from build123d import *
from OCP.BRepFilletAPI import BRepFilletAPI_MakeChamfer

# Parameters (mm, degrees)
PROFILE_SKETCH_W         = 14.3
PROFILE_SKETCH_H         = 6.7
PROFILE_SKETCH_W_2       = 10.1
PROFILE_SKETCH_H_2       = 2.5
PROFILE_EXTRUDE_DEPTH    = 15
OUTSIDE_CORNER_FILLETS_R = 1.5
END_1_CHAMFER_SIZE       = 1
END_1_CHAMFER_SIZE2      = 0.363970234
END_2_CHAMFER_SIZE       = 1
END_2_CHAMFER_SIZE2      = 0.363970234
TRANSITION_FILLETS_R     = 2.5


with BuildPart() as part:
    # Profile Sketch → Profile Extrude (new body)
    with BuildSketch(Plane.XY):
        Rectangle(PROFILE_SKETCH_W, PROFILE_SKETCH_H)
        Rectangle(PROFILE_SKETCH_W_2, PROFILE_SKETCH_H_2, mode=Mode.SUBTRACT)
    extrude(amount=PROFILE_EXTRUDE_DEPTH)

    # Outside Corner Fillets
    outside_corner_fillets_edges = [part.edges().sort_by_distance(p)[0] for p in [
        (7.15, -3.35, 7.5),
        (-7.15, -3.35, 7.5),
        (-7.15, 3.35, 7.5),
        (7.15, 3.35, 7.5),
    ]]
    fillet(outside_corner_fillets_edges, radius=OUTSIDE_CORNER_FILLETS_R)

    # End 1 Chamfer: one chamfer whose edges measure the first distance from different faces: ONE call of the kernel's chamfer builder (chamfer() names one face for all edges)
    end_1_chamfer_edges_1 = [part.edges().sort_by_distance(p)[0] for p in [
        (5.05, 0, 15),
    ]]
    end_1_chamfer_side_1 = [part.faces().sort_by_distance(p)[0] for p in [
        (5.05, 0, 7.5),
    ]]
    end_1_chamfer_edges_2 = [part.edges().sort_by_distance(p)[0] for p in [
        (0, 1.25, 15),
    ]]
    end_1_chamfer_side_2 = [part.faces().sort_by_distance(p)[0] for p in [
        (0, 1.25, 7.5),
    ]]
    end_1_chamfer_edges_3 = [part.edges().sort_by_distance(p)[0] for p in [
        (-5.05, 0, 15),
    ]]
    end_1_chamfer_side_3 = [part.faces().sort_by_distance(p)[0] for p in [
        (-5.05, 0, 7.5),
    ]]
    end_1_chamfer_edges_4 = [part.edges().sort_by_distance(p)[0] for p in [
        (0, -1.25, 15),
    ]]
    end_1_chamfer_side_4 = [part.faces().sort_by_distance(p)[0] for p in [
        (0, -1.25, 7.5),
    ]]
    end_1_chamfer_edges_5 = [part.edges().sort_by_distance(p)[0] for p in [
        (0, 3.35, 0),
    ]]
    end_1_chamfer_side_5 = [part.faces().sort_by_distance(p)[0] for p in [
        (0, 3.35, 7.5),
    ]]
    end_1_chamfer_edges_6 = [part.edges().sort_by_distance(p)[0] for p in [
        (7.15, 0, 0),
    ]]
    end_1_chamfer_side_6 = [part.faces().sort_by_distance(p)[0] for p in [
        (7.15, 0, 7.5),
    ]]
    end_1_chamfer_edges_7 = [part.edges().sort_by_distance(p)[0] for p in [
        (0, -3.35, 0),
    ]]
    end_1_chamfer_side_7 = [part.faces().sort_by_distance(p)[0] for p in [
        (0, -3.35, 7.5),
    ]]
    end_1_chamfer_edges_8 = [part.edges().sort_by_distance(p)[0] for p in [
        (-7.15, 0, 0),
    ]]
    end_1_chamfer_side_8 = [part.faces().sort_by_distance(p)[0] for p in [
        (-7.15, 0, 7.5),
    ]]
    end_1_chamfer_edges_9 = [part.edges().sort_by_distance(p)[0] for p in [
        (-6.710660172, -2.910660172, 0),
    ]]
    end_1_chamfer_side_9 = [part.faces().sort_by_distance(p)[0] for p in [
        (-6.710660172, -2.910660172, 7.5),
    ]]
    end_1_chamfer_edges_10 = [part.edges().sort_by_distance(p)[0] for p in [
        (-6.710660172, 2.910660172, 0),
    ]]
    end_1_chamfer_side_10 = [part.faces().sort_by_distance(p)[0] for p in [
        (-6.710660172, 2.910660172, 7.5),
    ]]
    end_1_chamfer_edges_11 = [part.edges().sort_by_distance(p)[0] for p in [
        (6.710660172, -2.910660172, 0),
    ]]
    end_1_chamfer_side_11 = [part.faces().sort_by_distance(p)[0] for p in [
        (6.710660172, -2.910660172, 7.5),
    ]]
    end_1_chamfer_edges_12 = [part.edges().sort_by_distance(p)[0] for p in [
        (6.710660172, 2.910660172, 0),
    ]]
    end_1_chamfer_side_12 = [part.faces().sort_by_distance(p)[0] for p in [
        (6.710660172, 2.910660172, 7.5),
    ]]
    end_1_chamfer = BRepFilletAPI_MakeChamfer(part.part.solid().wrapped)
    for e in end_1_chamfer_edges_1:
        end_1_chamfer.Add(END_1_CHAMFER_SIZE, END_1_CHAMFER_SIZE2, e.wrapped, end_1_chamfer_side_1[0].wrapped)  # the first distance lies on this face
    for e in end_1_chamfer_edges_2:
        end_1_chamfer.Add(END_1_CHAMFER_SIZE, END_1_CHAMFER_SIZE2, e.wrapped, end_1_chamfer_side_2[0].wrapped)  # the first distance lies on this face
    for e in end_1_chamfer_edges_3:
        end_1_chamfer.Add(END_1_CHAMFER_SIZE, END_1_CHAMFER_SIZE2, e.wrapped, end_1_chamfer_side_3[0].wrapped)  # the first distance lies on this face
    for e in end_1_chamfer_edges_4:
        end_1_chamfer.Add(END_1_CHAMFER_SIZE, END_1_CHAMFER_SIZE2, e.wrapped, end_1_chamfer_side_4[0].wrapped)  # the first distance lies on this face
    for e in end_1_chamfer_edges_5:
        end_1_chamfer.Add(END_1_CHAMFER_SIZE, END_1_CHAMFER_SIZE2, e.wrapped, end_1_chamfer_side_5[0].wrapped)  # the first distance lies on this face
    for e in end_1_chamfer_edges_6:
        end_1_chamfer.Add(END_1_CHAMFER_SIZE, END_1_CHAMFER_SIZE2, e.wrapped, end_1_chamfer_side_6[0].wrapped)  # the first distance lies on this face
    for e in end_1_chamfer_edges_7:
        end_1_chamfer.Add(END_1_CHAMFER_SIZE, END_1_CHAMFER_SIZE2, e.wrapped, end_1_chamfer_side_7[0].wrapped)  # the first distance lies on this face
    for e in end_1_chamfer_edges_8:
        end_1_chamfer.Add(END_1_CHAMFER_SIZE, END_1_CHAMFER_SIZE2, e.wrapped, end_1_chamfer_side_8[0].wrapped)  # the first distance lies on this face
    for e in end_1_chamfer_edges_9:
        end_1_chamfer.Add(END_1_CHAMFER_SIZE, END_1_CHAMFER_SIZE2, e.wrapped, end_1_chamfer_side_9[0].wrapped)  # the first distance lies on this face
    for e in end_1_chamfer_edges_10:
        end_1_chamfer.Add(END_1_CHAMFER_SIZE, END_1_CHAMFER_SIZE2, e.wrapped, end_1_chamfer_side_10[0].wrapped)  # the first distance lies on this face
    for e in end_1_chamfer_edges_11:
        end_1_chamfer.Add(END_1_CHAMFER_SIZE, END_1_CHAMFER_SIZE2, e.wrapped, end_1_chamfer_side_11[0].wrapped)  # the first distance lies on this face
    for e in end_1_chamfer_edges_12:
        end_1_chamfer.Add(END_1_CHAMFER_SIZE, END_1_CHAMFER_SIZE2, e.wrapped, end_1_chamfer_side_12[0].wrapped)  # the first distance lies on this face
    add(Compound.cast(end_1_chamfer.Shape()), mode=Mode.REPLACE)

    # End 2 Chamfer: one chamfer whose edges measure the first distance from different faces: ONE call of the kernel's chamfer builder (chamfer() names one face for all edges)
    end_2_chamfer_edges_1 = [part.edges().sort_by_distance(p)[0] for p in [
        (5.05, 0, 0),
    ]]
    end_2_chamfer_side_1 = [part.faces().sort_by_distance(p)[0] for p in [
        (5.05, 0, 7),
    ]]
    end_2_chamfer_edges_2 = [part.edges().sort_by_distance(p)[0] for p in [
        (0, 1.25, 0),
    ]]
    end_2_chamfer_side_2 = [part.faces().sort_by_distance(p)[0] for p in [
        (0, 1.25, 7),
    ]]
    end_2_chamfer_edges_3 = [part.edges().sort_by_distance(p)[0] for p in [
        (-5.05, 0, 0),
    ]]
    end_2_chamfer_side_3 = [part.faces().sort_by_distance(p)[0] for p in [
        (-5.05, 0, 7),
    ]]
    end_2_chamfer_edges_4 = [part.edges().sort_by_distance(p)[0] for p in [
        (0, -1.25, 0),
    ]]
    end_2_chamfer_side_4 = [part.faces().sort_by_distance(p)[0] for p in [
        (0, -1.25, 7),
    ]]
    end_2_chamfer_edges_5 = [part.edges().sort_by_distance(p)[0] for p in [
        (0, 3.35, 15),
    ]]
    end_2_chamfer_side_5 = [part.faces().sort_by_distance(p)[0] for p in [
        (0, 3.35, 8),
    ]]
    end_2_chamfer_edges_6 = [part.edges().sort_by_distance(p)[0] for p in [
        (7.15, 0, 15),
    ]]
    end_2_chamfer_side_6 = [part.faces().sort_by_distance(p)[0] for p in [
        (7.15, 0, 8),
    ]]
    end_2_chamfer_edges_7 = [part.edges().sort_by_distance(p)[0] for p in [
        (-7.15, 0, 15),
    ]]
    end_2_chamfer_side_7 = [part.faces().sort_by_distance(p)[0] for p in [
        (-7.15, 0, 8),
    ]]
    end_2_chamfer_edges_8 = [part.edges().sort_by_distance(p)[0] for p in [
        (0, -3.35, 15),
    ]]
    end_2_chamfer_side_8 = [part.faces().sort_by_distance(p)[0] for p in [
        (0, -3.35, 8),
    ]]
    end_2_chamfer_edges_9 = [part.edges().sort_by_distance(p)[0] for p in [
        (-6.710660172, -2.910660172, 15),
    ]]
    end_2_chamfer_side_9 = [part.faces().sort_by_distance(p)[0] for p in [
        (-6.710660172, -2.910660172, 8),
    ]]
    end_2_chamfer_edges_10 = [part.edges().sort_by_distance(p)[0] for p in [
        (-6.710660172, 2.910660172, 15),
    ]]
    end_2_chamfer_side_10 = [part.faces().sort_by_distance(p)[0] for p in [
        (-6.710660172, 2.910660172, 8),
    ]]
    end_2_chamfer_edges_11 = [part.edges().sort_by_distance(p)[0] for p in [
        (6.710660172, -2.910660172, 15),
    ]]
    end_2_chamfer_side_11 = [part.faces().sort_by_distance(p)[0] for p in [
        (6.710660172, -2.910660172, 8),
    ]]
    end_2_chamfer_edges_12 = [part.edges().sort_by_distance(p)[0] for p in [
        (6.710660172, 2.910660172, 15),
    ]]
    end_2_chamfer_side_12 = [part.faces().sort_by_distance(p)[0] for p in [
        (6.710660172, 2.910660172, 8),
    ]]
    end_2_chamfer = BRepFilletAPI_MakeChamfer(part.part.solid().wrapped)
    for e in end_2_chamfer_edges_1:
        end_2_chamfer.Add(END_2_CHAMFER_SIZE, END_2_CHAMFER_SIZE2, e.wrapped, end_2_chamfer_side_1[0].wrapped)  # the first distance lies on this face
    for e in end_2_chamfer_edges_2:
        end_2_chamfer.Add(END_2_CHAMFER_SIZE, END_2_CHAMFER_SIZE2, e.wrapped, end_2_chamfer_side_2[0].wrapped)  # the first distance lies on this face
    for e in end_2_chamfer_edges_3:
        end_2_chamfer.Add(END_2_CHAMFER_SIZE, END_2_CHAMFER_SIZE2, e.wrapped, end_2_chamfer_side_3[0].wrapped)  # the first distance lies on this face
    for e in end_2_chamfer_edges_4:
        end_2_chamfer.Add(END_2_CHAMFER_SIZE, END_2_CHAMFER_SIZE2, e.wrapped, end_2_chamfer_side_4[0].wrapped)  # the first distance lies on this face
    for e in end_2_chamfer_edges_5:
        end_2_chamfer.Add(END_2_CHAMFER_SIZE, END_2_CHAMFER_SIZE2, e.wrapped, end_2_chamfer_side_5[0].wrapped)  # the first distance lies on this face
    for e in end_2_chamfer_edges_6:
        end_2_chamfer.Add(END_2_CHAMFER_SIZE, END_2_CHAMFER_SIZE2, e.wrapped, end_2_chamfer_side_6[0].wrapped)  # the first distance lies on this face
    for e in end_2_chamfer_edges_7:
        end_2_chamfer.Add(END_2_CHAMFER_SIZE, END_2_CHAMFER_SIZE2, e.wrapped, end_2_chamfer_side_7[0].wrapped)  # the first distance lies on this face
    for e in end_2_chamfer_edges_8:
        end_2_chamfer.Add(END_2_CHAMFER_SIZE, END_2_CHAMFER_SIZE2, e.wrapped, end_2_chamfer_side_8[0].wrapped)  # the first distance lies on this face
    for e in end_2_chamfer_edges_9:
        end_2_chamfer.Add(END_2_CHAMFER_SIZE, END_2_CHAMFER_SIZE2, e.wrapped, end_2_chamfer_side_9[0].wrapped)  # the first distance lies on this face
    for e in end_2_chamfer_edges_10:
        end_2_chamfer.Add(END_2_CHAMFER_SIZE, END_2_CHAMFER_SIZE2, e.wrapped, end_2_chamfer_side_10[0].wrapped)  # the first distance lies on this face
    for e in end_2_chamfer_edges_11:
        end_2_chamfer.Add(END_2_CHAMFER_SIZE, END_2_CHAMFER_SIZE2, e.wrapped, end_2_chamfer_side_11[0].wrapped)  # the first distance lies on this face
    for e in end_2_chamfer_edges_12:
        end_2_chamfer.Add(END_2_CHAMFER_SIZE, END_2_CHAMFER_SIZE2, e.wrapped, end_2_chamfer_side_12[0].wrapped)  # the first distance lies on this face
    add(Compound.cast(end_2_chamfer.Shape()), mode=Mode.REPLACE)

    # Transition Fillets
    transition_fillets_edges = [part.edges().sort_by_distance(p)[0] for p in [
        (0, -3.35, 14),
        (6.710660172, -2.910660172, 14),
        (-6.710660172, -2.910660172, 14),
        (7.15, 0, 14),
        (-7.15, 0, 14),
        (6.710660172, 2.910660172, 14),
        (-6.710660172, 2.910660172, 14),
        (0, 3.35, 14),
        (5.05, 0, 14),
        (0, 1.25, 14),
        (-5.05, 0, 14),
        (0, -1.25, 14),
        (0, -3.35, 1),
        (6.710660172, -2.910660172, 1),
        (-6.710660172, -2.910660172, 1),
        (7.15, 0, 1),
        (-7.15, 0, 1),
        (6.710660172, 2.910660172, 1),
        (-6.710660172, 2.910660172, 1),
        (0, 3.35, 1),
        (5.05, 0, 1),
        (0, 1.25, 1),
        (-5.05, 0, 1),
        (0, -1.25, 1),
    ]]
    fillet(transition_fillets_edges, radius=TRANSITION_FILLETS_R)


solid = part.part
Geometry: final body of the model. Coordinates: model frame, mm. A direction names the side the tool comes from. Give positions to 0.01 mm unless a question says otherwise; leave off trailing zeros. Loops run counter-clockwise (first coordinate to the right, second up) from the corner with the lowest first, then second, coordinate; pieces in that order, holes last. Notation, with made-up numbers: (12, 57.25) - (23, 57.25) arc R14 ccw to (23, 62.25) - close; hole circle Ø6 at (-33.5, -40). An arc over 180 degrees is marked (long way). Answer as CSV lines item,"result". Start each with the question number.
1. Reachability of faces 1 (the face through (0, 1.25, 7)), 2 (the face through (-6.52, 2.7, 14.78)), 3 (the face through (0.07, 1.29, 14)) from +Z, -Z, +X, -X, +Y, -Y: full face, straight path, thin tool, end or side. Return the list, or none.
2. Section B-B, the plane y = -1. Return loops of the section in (x, z).
3. Draft query along X for faces 4 (the face through (-5.09, 0.02, 14)), 5 (the face through (7.15, 0, 7)), 6 (the face through (0, -3.35, 7)), 7 (the face through (5.09, 0.02, 1)). Return one class per face: released by +X, released by -X, zero draft, split by the parting line, or undercut.
4. Ray query, L1, parallel to Y at x = 0.5, z = 3.5; L2, parallel to X at y = 1, z = 12; L3, parallel to Y at x = 2.25, z = 14. Return the intervals inside material, ascending.
5. Section A-A, the plane x = -3.75. Return loops of the section in (y, z), plus the area to 3 significant figures.
6. Section C-C, the plane z = 7.75. Return loops of the section in (x, y), plus the area to 3 significant figures.
Answers:
1,face 1,"+Z, -Z"
1,face 2,"+Z, -X, +Y"
1,face 3,"+Z"
2,outline,"(-7.15, 1.44) arc R2.5 ccw to (-7, 0.59) - (-6.79, 0) - (-5.41, 0) - (-5.2, 0.59) arc R2.5 ccw to (-5.05, 1.44) - (-5.05, 13.56) arc R2.5 ccw to (-5.2, 14.41) - (-5.41, 15) - (-6.79, 15) - (-7, 14.41) arc R2.5 ccw to (-7.15, 13.56) - close; (5.05, 1.44) arc R2.5 ccw to (5.2, 0.59) - (5.41, 0) - (6.79, 0) - (7, 0.59) arc R2.5 ccw to (7.15, 1.44) - (7.15, 13.56) arc R2.5 ccw to (7, 14.41) - (6.79, 15) - (5.41, 15) - (5.2, 14.41) arc R2.5 ccw to (5.05, 13.56) - close"
3,face 4,"undercut"
3,face 5,"released by +X"
3,face 6,"zero draft"
3,face 7,"undercut"
4,L1,"y = -3.35 to -1.25, 1.25 to 3.35"
4,L2,"x = -7.15 to -5.05, 5.05 to 7.15"
4,L3,"y = -3.31 to -1.29, 1.29 to 3.31"
5,outline,"(-3.35, 1.44) arc R2.5 ccw to (-3.2, 0.59) - (-2.99, 0) - (-1.61, 0) - (-1.4, 0.59) arc R2.5 ccw to (-1.25, 1.44) - (-1.25, 13.56) arc R2.5 ccw to (-1.4, 14.41) - (-1.61, 15) - (-2.99, 15) - (-3.2, 14.41) arc R2.5 ccw to (-3.35, 13.56) - close; (1.25, 1.44) arc R2.5 ccw to (1.4, 0.59) - (1.61, 0) - (2.99, 0) - (3.2, 0.59) arc R2.5 ccw to (3.35, 1.44) - (3.35, 13.56) arc R2.5 ccw to (3.2, 14.41) - (2.99, 15) - (1.61, 15) - (1.4, 14.41) arc R2.5 ccw to (1.25, 13.56) - close"
5,area,"61.5 mm2"
6,outline,"(-7.15, -1.85) arc R1.5 ccw to (-5.65, -3.35) - (5.65, -3.35) arc R1.5 ccw to (7.15, -1.85) - (7.15, 1.85) arc R1.5 ccw to (5.65, 3.35) - (-5.65, 3.35) arc R1.5 ccw to (-7.15, 1.85) - close; hole (-5.05, -1.25) - (5.05, -1.25) - (5.05, 1.25) - (-5.05, 1.25) - close"
6,area,"68.6 mm2"
